Geometry: final body of the model. Coordinates: model frame, mm. Face numbers are marked on the shaded views. Give positions to 0.01 mm unless a question says otherwise; leave off trailing zeros. Order: outer loops, then holes, each group sorted by start corner. A loop starts at its lowest first (then second) coordinate and runs counter-clockwise, first axis right, second up. Notation, with made-up numbers: (87.5, 74.5) - (113.5, 74.5) arc R24 ccw to (113.5, 97.5) - close; hole circle Ø10 at (56.25, 68.5). An arc over 180 degrees is marked (long way). One line per item, written item: value.
```python
from build123d import *

# Parameters (mm, degrees)
F0_R     = 59.69
F1_DEPTH = 6.35
F2_R     = 59.69
F2_R_2   = 57.277
F3_DEPTH = 19.05
F4_R     = 4.7625
F5_DEPTH = 25.4


# Not quite as in the source:
# - a feature names something its author has since deleted; it is built from what else it names


with BuildPart() as f1:
    # F0 (on Top) → F1 (new body)
    with BuildSketch(Plane.XY):
        Circle(F0_R)
    extrude(amount=F1_DEPTH)

    # F2 (on face) → F3 (join)
    with BuildSketch(Plane.XY.offset(6.35)):
        Circle(F2_R)
        Circle(F2_R_2, mode=Mode.SUBTRACT)
    extrude(amount=F3_DEPTH)

    # F4 (on face) → F5 (cut)
    with BuildSketch(Plane.XY.offset(6.35)):
        Circle(F4_R)
    extrude(amount=-F5_DEPTH, mode=Mode.SUBTRACT)


solid = f1.part
```
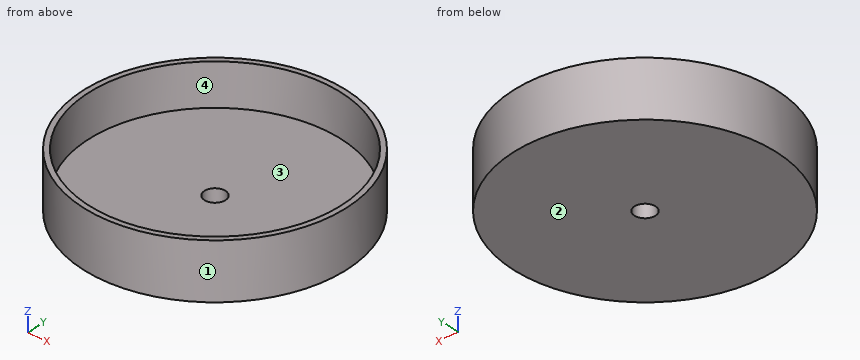
1) Section D-D, the plane z = 13.75. Return loops of the section in (x, y), then the cut area to 3 significant figures.
Answers below:
outline: circle Ø119.38 at (0, 0); hole circle Ø114.55 at (0, 0)
area: 887 mm^2
2) Material intervals for line 1 along Y through (x, z) = (0, 4.5); line 2 along Y through (x, z) = (0, 13.5); line 3 along Z through (x, y) = (40.5, 21), sorted ascending.
Answers below:
line 1: -59.69 to -4.76, 4.76 to 59.69
line 2: -59.69 to -57.28, 57.28 to 59.69
line 3: 0 to 6.35
3) Mould query, pull axis Y, two halves, no side actions, for the marked faces 1, 2, 3 and 4. Classes: released by +Y, released by -Y, zero draft, split by the parting line, or undercut.
Answers below:
face 1: split by the parting line
face 2: zero draft
face 3: undercut
face 4: undercut
4) Section C-C, the plane x = -40.5. Return loops of the section in (y, z).
Answers below:
outline: (-43.85, 0) - (43.85, 0) - (43.85, 25.4) - (40.5, 25.4) - (40.5, 6.35) - (-40.5, 6.35) - (-40.5, 25.4) - (-43.85, 25.4) - close
5) Section A-A, the plane x = 0. Return loops of the section in (y, z).
Answers below:
outline: (-59.69, 0) - (-4.76, 0) - (-4.76, 6.35) - (-57.28, 6.35) - (-57.28, 25.4) - (-59.69, 25.4) - close; (4.76, 0) - (59.69, 0) - (59.69, 25.4) - (57.28, 25.4) - (57.28, 6.35) - (4.76, 6.35) - close
6) First-contact query: pin 1 (1 mm diameter, centred on x = 7, y = 10.5, fed in from -Z); pin 2 (1.5 mm diameter, centred on x = 12.5, y = 31, fed in from +Z); pin 3 (1 mm diameter, centred on x = -16, z = 13, fed in from -Y); pin 4 (12 mm diameter, centred on x = -20.5, z = 22, fed in from +Y). Flat tips, straight axial feed; report the tip coordinate or a pass-through.
Answers below:
pin 1: z = 0
pin 2: z = 6.35
pin 3: y = -57.64
pin 4: y = 57.9
